```python
from build123d import *

# Parameters (mm, degrees)
SKETCH1_W                = 14.75
SKETCH1_H                = 9.75
BOSS_EXTRUDE1_DEPTH      = 50
BOSS_EXTRUDE2_DEPTH      = 18.875
BOSS_EXTRUDE2_DEPTH_BACK = 18.875


with BuildPart() as part:
    # Sketch1 → Boss-Extrude1 (new body)
    with BuildSketch(Plane(origin=(0, 0, 0), x_dir=(1, 0, 0), z_dir=(0, 1, 0))):
        with Locations((0, -0.125)):
            Rectangle(SKETCH1_W, SKETCH1_H)
    extrude(amount=BOSS_EXTRUDE1_DEPTH)

    # Sketch3 → Boss-Extrude2 (add, two sides: drawn at the far end of the back side and taken through both)
    with BuildSketch(Plane(origin=(0, 0, 0), x_dir=(0, 0, -1), z_dir=(1, 0, 0)).offset(-BOSS_EXTRUDE2_DEPTH_BACK)):
        Polygon((-10.25, 20), (-5.25, 20), (9.75, 20), (9.75, 50), (-10.25, 50), align=None)
    extrude(amount=BOSS_EXTRUDE2_DEPTH + BOSS_EXTRUDE2_DEPTH_BACK)


solid = part.part
```
Work out the finished part from the listing and answer in its coordinate system (mm). A direction names the side the tool comes from. Give positions to 0.01 mm unless a question says otherwise; leave off trailing zeros. Loops run counter-clockwise (first coordinate to the right, second up) from the corner with the lowest first, then second, coordinate; pieces in that order, holes last. Notation, with made-up numbers: M -12.75,77.5 L 1.25,77.5 A27 cw 1.25,99.5 Z; hole C -31,-23 d5. An arc over 180 degrees is marked long. One line per item, written item: value. Start each with the question number.
1. Determine the mould class of faces 1 (the face through (0, 20, 7)), 2 (the face through (-18.875, 35, 0)), 3 (the face through (7.375, 10, 0)) for opening direction X: released by +X, released by -X, zero draft, split by the parting line, or undercut.
2. Find the intervals of material crossed by probe 1 along Y at (x, z) = (-11, -0.5); probe 2 along X at (y, z) = (6, 3.25) (3 decimals); probe 3 along Z at (x, y) = (3.5, 12), in increasing order.
3. Each of these flat-tipped pins is pushed along its axis until it touches: P1, Ø7.5, axis at x = 3.5, y = 13, coming from the +Z side; P2, Ø4.5, axis at x = -2, y = 12.5, coming from the -Z side; P3, Ø10.5, axis at y = 13, z = -0.5, coming from the +X side (3 decimals). Where does it stop, or does it pass through?
4. Find section A-A (z = 3). Give the vertices of the cut face in (x, y) (3 decimals), and give its area (3 significant figures).
5. Which of the six approach directions +Z, -Z, +X, -X, +Y, -Y give full straight-line access (tool end or side, diameter ignored) to faces 4 (the face through (0, 10, -4.75)), 5 (the face through (-7.375, 10, 0)), 6 (the face through (0, 10, 5))?
6. Find section B-B (x = -3). Give the vertices of the cut face in (y, z).
7. Find section D-D (x = -10.5). Give the vertices of the cut face in (y, z).
8. Find section C-C (y = 14). Give the vertices of the cut face in (x, z) (3 decimals).
Reported:
1. face 1: zero draft
1. face 2: released by -X
1. face 3: released by +X
2. probe 1: y = 20 to 50
2. probe 2: x = -7.375 to 7.375
2. probe 3: z = -4.75 to 5
3. P1: stops at z = 5
3. P2: stops at z = -4.75
3. P3: stops at x = 7.375
4. outline: M -18.875,20 L -7.375,20 L -7.375,0 L 7.375,0 L 7.375,20 L 18.875,20 L 18.875,50 L -18.875,50 Z
4. area: 1,430 mm²
5. face 4: -Z, +X, -X, -Y
5. face 5: +Z, -Z, -X, -Y
5. face 6: +Z, +X, -X, -Y
6. outline: M 0,-4.75 L 20,-4.75 L 20,-9.75 L 50,-9.75 L 50,10.25 L 20,10.25 L 20,5 L 0,5 Z
7. outline: M 20,-9.75 L 50,-9.75 L 50,10.25 L 20,10.25 Z
8. outline: M -7.375,-4.75 L 7.375,-4.75 L 7.375,5 L -7.375,5 Z
